from build123d import *

# Parameters (mm, degrees)
F1_DEPTH = 12.7
F2_R     = 1.5875
F4_D     = 6.35


with BuildPart() as f1:
    # F0 (on Top) → F1 (new body)
    with BuildSketch(Plane.XY):
        with BuildLine():
            ThreePointArc((3.175, 15.5542598667), (15.875, 0), (3.175, -15.5542598667))
            Line((3.175, -15.5542598667), (3.175, -18.7292598667))
            ThreePointArc((3.175, -18.7292598667), (4.7801025689, -18.3908223826), (6.35, -17.9150953144))
            ThreePointArc((6.35, -17.9150953144), (19.05, 0), (6.35, 17.9150953144))
            ThreePointArc((6.35, 17.9150953144), (4.7801025689, 18.3908223826), (3.175, 18.7292598667))
            Line((3.175, 18.7292598667), (3.175, 15.5542598667))
        make_face()
        with BuildLine():
            Line((3.175, 28.575), (3.175, 18.7292598667))
            ThreePointArc((3.175, 18.7292598667), (4.7801025689, 18.3908223826), (6.35, 17.9150953144))
            Line((6.35, 17.9150953144), (6.35, 28.575))
            Line((6.35, 28.575), (3.175, 28.575))
        make_face()
        with BuildLine():
            ThreePointArc((6.35, -17.9150953144), (4.7801025689, -18.3908223826), (3.175, -18.7292598667))
            Line((3.175, -18.7292598667), (3.175, -28.575))
            Line((3.175, -28.575), (6.35, -28.575))
            Line((6.35, -28.575), (6.35, -17.9150953144))
        make_face()
    extrude(amount=F1_DEPTH)

    # F2
    f2_edges = [f1.edges().sort_by_distance(p)[0] for p in [
        (4.7625, 28.575, 12.7),
        (4.7625, 28.575, 0),
        (4.7625, -28.575, 0),
        (4.7625, -28.575, 12.7),
    ]]
    fillet(f2_edges, radius=F2_R)

    # F4 (through all)
    with Locations(Plane.YZ.offset(6.35)):
        with Locations((-23.2450476572, 6.35), (23.2450476572, 6.35)):
            Hole(F4_D / 2)


solid = f1.part
Geometry: final body of the model. Coordinates: model frame, mm. A direction names the side the tool comes from. Give positions to 0.01 mm unless a question says otherwise; leave off trailing zeros. Write each loop counter-clockwise with the first axis right and the second up, starting at its lowest first coordinate (ties: lowest second). Pieces come first, ordered by that corner, then holes. Notation, with made-up numbers: M 4.25,-9 L 31.25,-9 A16 cw 31.25,9 Z; hole C -1,1 d3. An arc over 180 degrees is marked long. Answer in a Markdown table with one row per item. Add a question column.
(1) Reachability of faces 1 (the flat face through (6.35, -19.8, 6.3)), 2 (the cylindrical face through (4.74, -26.273, 7.304)) from +Z, -Z, +X, -X, +Y, -Y: full face, straight path, thin tool, end or side. Return the list, or none.
(2) Section B-B on z = 5.5. Return loops of the section in (x, y) (3 decimals).
(3) Mould query, pull axis Y, two halves, no side actions, for faces 3 (the cylindrical face through (4.74, 20.217, 7.304)), 4 (the cylindrical face through (4.785, -28.122, 0.477)), 5 (the flat face through (6.35, 19.6, 6.3)). Classes: +Y half, -Y half, draft (parallel to the pull), parting line (faces both ways), or undercut.
(4) Section D-D on z = 7.75. Return loops of the section in (x, y) (3 decimals).
(5) First-contact query: pin 1 (6 mm diameter, centred on x = 14.5, z = 2, fed in from +Y); pin 2 (5 mm diameter, centred on x = 13, z = 3, fed in from -Y); pin 3 (2 mm diameter, centred on y = -10, z = 4, fed in from +X). Flat tips, straight axial feed; report the tip coordinate or a pass-through.
(6) Section C-C on y = -23.5. Return loops of the section in (x, z) (3 decimals).
(7) Ray query, line 1 (Z direction, x = 5.75, y = 25); line 2 (X direction, y = 23, z = 1.5) (3 decimals); line 3 (Y direction, x = 13.25, z = 9.25). Return the intervals inside material, ascending.
(8) Section A-A on x = 8. Return loops of the section in (y, z).
Result set:
| question | item | result |
|---|---|---|
| 1 | face 1 | +Z, -Z, +X, -Y |
| 1 | face 2 | +X, -X |
| 2 | outline | M 3.175,-28.575 L 6.35,-28.575 L 6.35,-26.304 L 3.175,-26.304 Z; M 3.175,-20.186 L 6.35,-20.186 L 6.35,-17.915 A18.986 ccw 6.35,17.915 L 6.35,20.186 L 3.175,20.186 L 3.175,15.554 A15.875 cw 3.175,-15.554 Z; M 3.175,26.304 L 6.35,26.304 L 6.35,28.575 L 3.175,28.575 Z |
| 3 | face 3 | undercut |
| 3 | face 4 | -Y half |
| 3 | face 5 | draft |
| 4 | outline | M 3.175,-28.575 L 6.35,-28.575 L 6.35,-26.095 L 3.175,-26.095 Z; M 3.175,-20.395 L 6.35,-20.395 L 6.35,-17.915 A18.986 ccw 6.35,17.915 L 6.35,20.395 L 3.175,20.395 L 3.175,15.554 A15.875 cw 3.175,-15.554 Z; M 3.175,26.095 L 6.35,26.095 L 6.35,28.575 L 3.175,28.575 Z |
| 5 | pin 1 | stops at y = 15.16 |
| 5 | pin 2 | stops at y = -15.86 |
| 5 | pin 3 | stops at x = 16.78 |
| 6 | outline | M 3.175,0 L 6.35,0 L 6.35,3.185 L 3.175,3.185 Z; M 3.175,9.515 L 6.35,9.515 L 6.35,12.7 L 3.175,12.7 Z |
| 7 | line 1 | z = 0 to 3.7, 9 to 12.7 |
| 7 | line 2 | x = 3.175 to 6.35 |
| 7 | line 3 | y = -13.66 to -8.74, 8.74 to 13.66 |
| 8 | outline | M -17.25,0 L -13.71,0 L -13.71,12.7 L -17.25,12.7 Z; M 13.71,0 L 17.25,0 L 17.25,12.7 L 13.71,12.7 Z |
